Source: CAD feature listing. Evaluate the final solid. Frame: model axes, mm. A direction names the side the tool comes from. Give positions to 0.01 mm unless a question says otherwise; leave off trailing zeros. Write each loop counter-clockwise with the first axis right and the second up, starting at its lowest first coordinate (ties: lowest second). Pieces come first, ordered by that corner, then holes. Notation, with made-up numbers: (-3.75, -10.5) -> (16.25, -10.5) arc R16 ccw to (16.25, 2.5) -> close; hole circle Ø4 at (-30.5, 34.5). An arc over 180 degrees is marked (long way). Write item = value, one per line.
from build123d import *

# Parameters (mm, degrees)
BOSS_EXTRUDE1_DEPTH = 35
SKETCH2_R           = 1.27
CUT_EXTRUDE1_DEPTH  = 35
CUT_EXTRUDE2_REACH  = 41.937
SKETCH3_W           = 10
SKETCH3_H           = 10
SKETCH4_R           = 2.049999964
CUT_EXTRUDE3_DEPTH  = 17.5
CUT_EXTRUDE5_START  = -7.95804
SKETCH6_R           = 2
CUT_EXTRUDE5_DEPTH  = 9.6
FILLET3_R           = 1
CUT_EXTRUDE6_START  = 8.64596
SKETCH6_3_R         = 2
CUT_EXTRUDE6_DEPTH  = 6.604
CUT_EXTRUDE7_START  = -14.986
CUT_EXTRUDE7_DEPTH  = 14.986
CUT_EXTRUDE8_DEPTH  = 31.496
SKETCH9_R           = 1.5
CUT_EXTRUDE9_DEPTH  = 14.224
CUT_EXTRUDE11_DEPTH = 6.048
SKETCH13_R          = 1.5
CUT_EXTRUDE12_DEPTH = 3
CUT_EXTRUDE13_START = -5.5
SKETCH15_R          = 2.75
CUT_EXTRUDE13_DEPTH = 7.572


with BuildPart() as part:
    # Sketch1 → Boss-Extrude1 (new body)
    with BuildSketch(Plane(origin=(0, 0, 0), x_dir=(1, 0, 0), z_dir=(0, 1, 0))):
        with BuildLine():
            Line((-2.958039892, 8.5), (2.958039892, 8.5))
            ThreePointArc((2.958039892, 8.5), (9, 0), (2.958039892, -8.5))
            Line((2.958039892, -8.5), (-2.958039892, -8.5))
            ThreePointArc((-2.958039892, -8.5), (-9, 0), (-2.958039892, 8.5))
        make_face()
    extrude(amount=BOSS_EXTRUDE1_DEPTH)

    # Sketch2 → Cut-Extrude1 (cut)
    with BuildSketch(Plane.XZ):
        with Locations(Location((0, -5, 0), (0, 0, 270))):
            Circle(SKETCH2_R)
        with Locations(Location((0, 5, 0), (0, 0, 270))):
            Circle(SKETCH2_R)
    extrude(amount=-CUT_EXTRUDE1_DEPTH, mode=Mode.SUBTRACT)

    # Cut-Extrude2: up to this face of the body (flat: up to its plane)
    cut_extrude2_end = Plane(part.part.faces().sort_by_distance((0, 17.5, 8.5))[0])
    # Sketch3 → Cut-Extrude2 (cut, up to the picked face)
    with BuildSketch(Plane(origin=(0, 0, -8.5), x_dir=(-1, 0, 0), z_dir=(0, 0, -1)), mode=Mode.PRIVATE) as cut_extrude2_sk1:
        with Locations((0, 5)):
            Rectangle(SKETCH3_W, SKETCH3_H)
    cut_extrude2_tool1 = split(extrude(cut_extrude2_sk1.sketch, amount=-CUT_EXTRUDE2_REACH, mode=Mode.PRIVATE), bisect_by=cut_extrude2_end, keep=Keep.BOTH, mode=Mode.PRIVATE)
    add(cut_extrude2_tool1.solids().sort_by(Axis((0, 5, -8.5), (0, 0, 1)))[0], mode=Mode.SUBTRACT)

    # Sketch4 → Cut-Extrude3 (cut, symmetric)
    with BuildSketch(Plane.ZY.offset(-5)):
        with Locations(Location((0, 5, 0), (0, 0, 270))):
            Circle(SKETCH4_R)
        with BuildLine():
            Line((-7.483314774, 10), (-5, 5))
            ThreePointArc((-5, 5), (0, 0), (5, 5))
            Line((5, 5), (8.5, 12.308552788))
            Line((8.5, 12.308552788), (9.857943437, -1.822240199))
            Line((9.857943437, -1.822240199), (-9.857943437, -1.822240199))
            Line((-9.857943437, -1.822240199), (-7.483314774, 10))
        make_face()
    extrude(amount=CUT_EXTRUDE3_DEPTH, both=True, mode=Mode.SUBTRACT)

    # Sketch6 → Cut-Extrude5 (cut)
    with BuildSketch(Plane.ZY.offset(2.958039892).offset(CUT_EXTRUDE5_START)):
        with BuildLine():
            Line((8.5, 21.219917379), (0, 25))
            ThreePointArc((0, 25), (-3.535533906, 26.464466094), (-5, 30))
            Line((-5, 30), (-6.755867779, 33.535330675))
            ThreePointArc((-6.755867779, 33.535330675), (-7.475170692, 34.449576169), (-8.5, 35))
            Line((-8.5, 35), (17.803004008, 42.886049022))
            Line((17.803004008, 42.886049022), (8.5, 21.219917379))
        make_face()
        with Locations((0, 30)):
            Circle(SKETCH6_R, mode=Mode.SUBTRACT)
    extrude(amount=-CUT_EXTRUDE5_DEPTH, mode=Mode.SUBTRACT)

    # Fillet3
    fillet3_edges = [part.edges().sort_by_distance(p)[0] for p in [
        (0, 10, -3.73),
        (0, 10, 6.27),
    ]]
    fillet(fillet3_edges, radius=FILLET3_R)

    # Sketch6<3> → Cut-Extrude6 (cut)
    with BuildSketch(Plane.ZY.offset(2.958039892).offset(CUT_EXTRUDE6_START)):
        with BuildLine():
            Line((8.5, 21.219917379), (0, 25))
            ThreePointArc((0, 25), (-3.535533906, 26.464466094), (-5, 30))
            Line((-5, 30), (-6.755867779, 33.535330675))
            ThreePointArc((-6.755867779, 33.535330675), (-7.475170692, 34.449576169), (-8.5, 35))
            Line((-8.5, 35), (17.803004008, 42.886049022))
            Line((17.803004008, 42.886049022), (8.5, 21.219917379))
        make_face()
        with Locations((0, 30)):
            Circle(SKETCH6_3_R, mode=Mode.SUBTRACT)
    extrude(amount=-CUT_EXTRUDE6_DEPTH, mode=Mode.SUBTRACT)

    # Sketch7 → Cut-Extrude7 (cut)
    with BuildSketch(Plane(origin=(5, 0, 0), x_dir=(0, 0, -1), z_dir=(1, 0, 0)).offset(CUT_EXTRUDE7_START)):
        with BuildLine():
            Line((5, 30), (6.755867779, 33.535330675))
            ThreePointArc((6.755867779, 33.535330675), (7.475170692, 34.449576169), (8.5, 35))
            Line((8.5, 35), (-8.341946035, 47.536710192))
            Line((-8.341946035, 47.536710192), (-13.168237897, 33.528506419))
            Line((-13.168237897, 33.528506419), (-10.04678731, 20.532036929))
            Line((-10.04678731, 20.532036929), (-4.915473018, 22.814012455))
            Line((-4.915473018, 22.814012455), (-4.915473018, 30.915491676))
            ThreePointArc((-4.915473018, 30.915491676), (0.459692783, 34.97882341), (5, 30))
        make_face()
    extrude(amount=CUT_EXTRUDE7_DEPTH, mode=Mode.SUBTRACT)

    # Sketch8 → Cut-Extrude8 (cut, symmetric)
    with BuildSketch(Plane.XZ.offset(-10)):
        with BuildLine():
            Line((0, 1.5), (0, -1.5))
            ThreePointArc((0, -1.5), (-3.5, -5), (0, -8.5))
            Line((0, -8.5), (-4.790142834, -16.013604782))
            Line((-4.790142834, -16.013604782), (34.96476625, -1.5))
            Line((34.96476625, -1.5), (-4.790142834, 15.219000931))
            Line((-4.790142834, 15.219000931), (0, 8.5))
            ThreePointArc((0, 8.5), (3.5, 5), (0, 1.5))
        make_face()
    extrude(amount=CUT_EXTRUDE8_DEPTH, both=True, mode=Mode.SUBTRACT)

    # Sketch9 → Cut-Extrude9 (cut)
    with BuildSketch(Plane(origin=(0, 0, 0), x_dir=(0, 0, -1), z_dir=(1, 0, 0))):
        with Locations((0, 16)):
            Circle(SKETCH9_R)
    extrude(amount=-CUT_EXTRUDE9_DEPTH, mode=Mode.SUBTRACT)

    # Sketch14 → Cut-Extrude11 (cut)
    with BuildSketch(Plane(origin=(0, 0, 0), x_dir=(0, 0, -1), z_dir=(1, 0, 0))):
        with BuildLine():
            Line((0, 12.5), (0, 19.5))
            ThreePointArc((0, 19.5), (-3.5, 16), (0, 12.5))
        make_face()
    extrude(amount=CUT_EXTRUDE11_DEPTH, mode=Mode.SUBTRACT)

    # Sketch13 → Cut-Extrude12 (cut)
    with BuildSketch(Plane(origin=(0, 0, 0), x_dir=(0, 0, -1), z_dir=(1, 0, 0))):
        with Locations((0, 30)):
            Circle(SKETCH13_R)
    extrude(amount=-CUT_EXTRUDE12_DEPTH, mode=Mode.SUBTRACT)

    # Sketch15 → Cut-Extrude13 (cut)
    with BuildSketch(Plane(origin=(0, 0, 0), x_dir=(0, 0, -1), z_dir=(1, 0, 0)).offset(CUT_EXTRUDE13_START)):
        with Locations((0, 16)):
            Circle(SKETCH15_R)
    extrude(amount=-CUT_EXTRUDE13_DEPTH, mode=Mode.SUBTRACT)


solid = part.part
1) Material intervals for L1, parallel to Y at x = -2.6, z = 0; L2, parallel to Y at x = -6.85, z = 0; L3, parallel to Y at x = -3.5, z = 0, sorted ascending.
Computed:
L1 = 10 to 14.5, 17.5 to 28.5, 31.5 to 35
L2 = 0 to 2.95, 7.05 to 13.25, 18.75 to 25, 28 to 32
L3 = 10 to 14.5, 17.5 to 35
2) Cut plane A-A (z = 0.5). Return the cut outline in (x, y), then the cut area to 3 significant figures.
Computed:
outline = (-8.99, 0.03) -> (-5, 0.03) -> (-5, 3.01) -> (-8.99, 3.01) -> close; (-8.99, 6.99) -> (-5, 6.99) -> (-5, 10) -> (0, 10) -> (0, 14.59) -> (-5.5, 14.59) -> (-5.5, 13.3) -> (-8.99, 13.3) -> close; (-8.99, 18.7) -> (-5.5, 18.7) -> (-5.5, 17.41) -> (0, 17.41) -> (0, 28.59) -> (-3, 28.59) -> (-3, 31.41) -> (0, 31.41) -> (0, 34.97) -> (-5, 34.97) -> (-5, 31.94) -> (-8.99, 31.94) -> (-8.99, 28.06) -> (-5, 28.06) -> (-5, 24.78) -> (-8.99, 24.78) -> close
area = 180 mm²
3) Contact query for flat-ended pins moving along their axis: pin 1 (1.9 mm diameter, centred on x = -2.5, y = 26.5, fed in from +Z); pin 2 (4 mm diameter, centred on x = -1, z = -2, fed in from -Y); pin 3 (1.5 mm diameter, centred on y = 20.5, z = 0, fed in from +X). Output: stop coordinate, or through.
Computed:
pin_1 = 4.92
pin_2 = 10
pin_3 = 0
4) Access query for faces 1 (the cylindrical face through (-7.23, 16.83, -2.62)), 2 (the flat face through (2, 27, 4.915)), 3 (the cylindrical face through (1.2, 16.1, 3.5)), 4 (the cylindrical face through (-3.675, 34.439, -7.463)), 5 (the flat face through (0, 33, 0)). Directions: +Z, -Z, +X, -X, +Y, -Y. A direction counts if a zero-diameter tool reaches every point of the face in a straight line with its end or side. Return the directions, or none.
Computed:
face_1 = -X
face_2 = +Z, +X, -X, +Y
face_3 = -Z, +X
face_4 = +X, -X, +Y
face_5 = -Z, +X, +Y, -Y
5) Draft query along Y for faces 6 (the cylindrical face through (-9, 30, 0)), 7 (the cylindrical face through (-1.479, 31.487, 0.195)), 8 (the flat face through (-5.983, 6.979, -5.983)). Return one class per face: pulls with the +Y half, pulls with the -Y half, needs draft (parallel to the pull), parting line crosses it, or undercut.
Computed:
face_6 = needs draft
face_7 = undercut
face_8 = pulls with the -Y half
6) Cut plane B-B (x = -6.75). Return the cut outline in (y, z).
Computed:
outline = (5, -5) -> (6.92, -5.95) -> (31.92, -5.95) -> (30, -5) arc R5 cw to (25, 0) -> (22.35, 5.95) -> (6.99, 5.95) -> (5, 5) arc R5 ccw to start; circle Ø4 at (30, 0); hole circle Ø4.1 at (5, 0); hole circle Ø5.5 at (16, 0)
7) Cut plane C-C (y = 32.5). Return the cut outline in (x, z).
Computed:
outline = (-6.48, -6.24) arc R9 ccw to (-2.96, -8.5) -> (0, -8.5) arc R3.5 cw to (-3.27, -6.24) -> close; (-5, -4.33) -> (-3.44, -4.33) arc R3.5 cw to (0, -1.5) -> (0, 1.5) arc R3.5 ccw to (3.44, 4.33) -> (1.08, 4.33) arc R1.27 cw to (-1.08, 4.33) -> (-5, 4.33) -> close
8) Cut plane D-D (z = -4.25). Return the cut outline in (x, y), then the cut area to 3 significant figures.
Computed:
outline = (-7.93, 2.37) -> (-5, 2.37) -> (-5, 10) -> (-3.42, 10) -> (-3.42, 32.63) -> (-5, 32.63) -> (-5, 27.37) -> (-7.93, 27.37) -> close
area = 109 mm²
